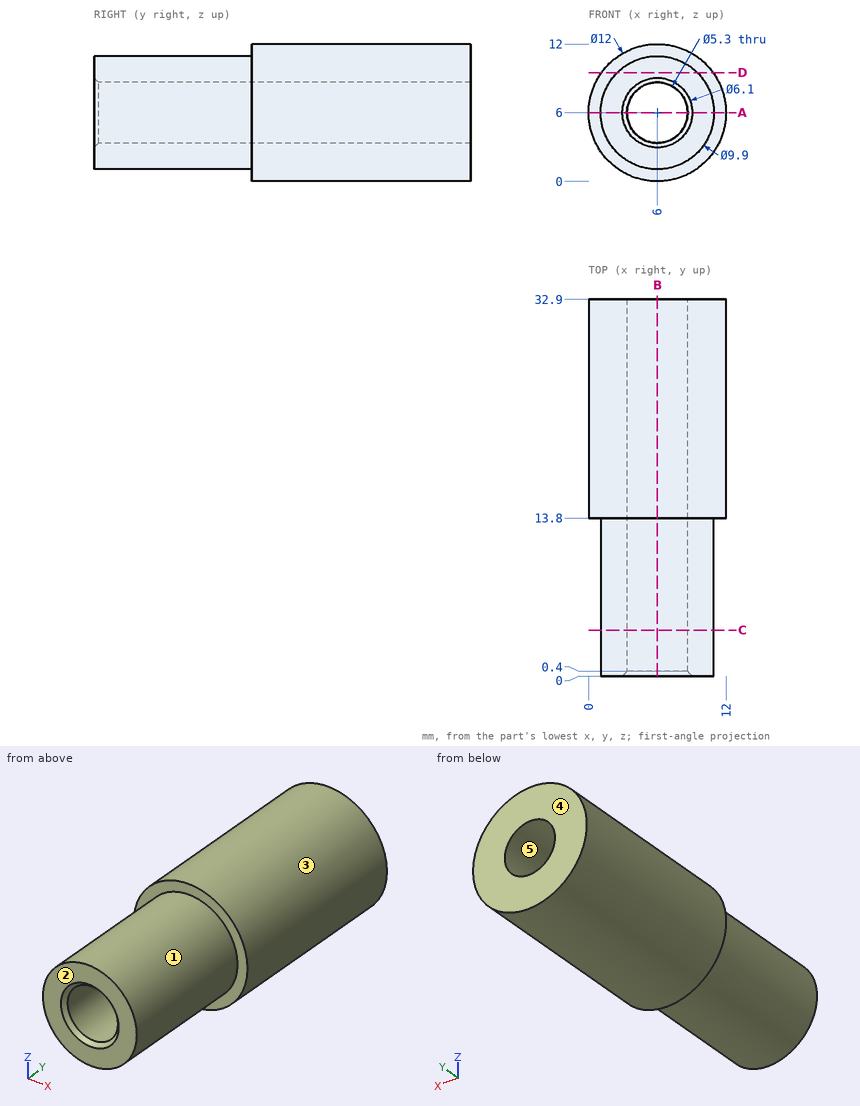
Answer from the drawing. Dimensions are ordinates in mm from the lowest x, y and z of the part. A direction names the side the tool comes from. Coordinates: 2 decimals unless noted, no trailing zeros. Loops run counter-clockwise (first coordinate to the right, second up) from the corner with the lowest first, then second, coordinate; pieces in that order, holes last. Notation, with made-up numbers: (64.25, 85.5) - (109.25, 85.5) arc R32 ccw to (109.25, 121.5) - close; hole circle Ø1 at (-24.75, 0). An arc over 180 degrees is marked (long way). Answer in a Markdown table with one row per item.
1. Find section A-A, the plane z = 6. Write down the section's boundary in (x, y), then the cut area to 3 significant figures.
Conclusion:
| item | result |
|---|---|
| outline | (0, 13.8) - (1.05, 13.8) - (1.05, 0) - (2.95, 0) - (3.35, 0.4) - (3.35, 32.9) - (0, 32.9) - close; (8.65, 0.4) - (9.05, 0) - (10.95, 0) - (10.95, 13.8) - (12, 13.8) - (12, 32.9) - (8.65, 32.9) - close |
| area | 191 mm² |
2. Determine the mould class of the marked faces 3, 4 and 5 for opening direction Z: +Z half, -Z half, draft (parallel to the pull), parting line (faces both ways), or undercut.
Conclusion:
| item | result |
|---|---|
| face 3 | parting line |
| face 4 | draft |
| face 5 | undercut |
3. Which of the six approach directions +Z, -Z, +X, -X, +Y, -Y give full straight-line access (tool end or side, diameter ignored) to the marked faces 1 and 2?
Conclusion:
| item | result |
|---|---|
| face 1 | -Y |
| face 2 | +Z, -Z, +X, -X, -Y |
4. Given pin 1 (5 mm diameter, centred on y = 19, z = 3, fed in from +X); pin 2 (6 mm diameter, centred on x = 1.5, y = 4.5, fed in from +Z); pin 3 (2 mm diameter, centred on y = 24.5, z = 3.5, fed in from -X), each flat-ended and moving along its own axis, determine where each tip first touches the part or whether it passes through.
Conclusion:
| item | result |
|---|---|
| pin 1 | stops at x = 11.98 |
| pin 2 | stops at z = 10.72 |
| pin 3 | stops at x = 0.19 |
5. Find section C-C, the plane y = 4. Write down the section's boundary in (x, z), then the cut area to 3 significant figures.
Conclusion:
| item | result |
|---|---|
| outline | circle Ø9.9 at (6, 6); hole circle Ø5.3 at (6, 6) |
| area | 54.9 mm² |
6. Straight lines are drawn through the part: line 1 (X direction, y = 11, z = 6); line 2 (Z direction, x = 6, y = 25.5). For each, find the intervals that lie inside material, in ascending order.
Conclusion:
| item | result |
|---|---|
| line 1 | x = 1.05 to 3.35, 8.65 to 10.95 |
| line 2 | z = 0 to 3.35, 8.65 to 12 |
7. Find section D-D, the plane z = 9.5. Write down the section's boundary in (x, y).
Conclusion:
| item | result |
|---|---|
| outline | (1.13, 13.8) - (2.5, 13.8) - (2.5, 0) - (9.5, 0) - (9.5, 13.8) - (10.87, 13.8) - (10.87, 32.9) - (1.13, 32.9) - close |
8. Find section B-B, the plane x = 6. Write down the section's boundary in (y, z), then the cut area to 3 significant figures.
Conclusion:
| item | result |
|---|---|
| outline | (0, 1.05) - (13.8, 1.05) - (13.8, 0) - (32.9, 0) - (32.9, 3.35) - (0.4, 3.35) - (0, 2.95) - close; (0, 9.05) - (0.4, 8.65) - (32.9, 8.65) - (32.9, 12) - (13.8, 12) - (13.8, 10.95) - (0, 10.95) - close |
| area | 191 mm² |
